Autodesk Inventor part; units mm, degrees
ref_plane "YZ Plane" through (0, 0, 0) normal (1, 0, 0) x (0, 1, 0)
ref_plane "XZ Plane" through (0, 0, 0) normal (0, 1, 0) x (-1, 0, 0)
ref_plane "XY Plane" through (0, 0, 0) normal (0, 0, 1) x (1, 0, 0)
sketch "Sketch1" plane through (0, 0, 0) normal (0, 0, 1) x (1, 0, 0)
  line L0 (-32, 32) -> (32, 32)
  line L1 (32, 32) -> (32, -32)
  line L2 (32, -32) -> (-32, -32)
  line L3 (-32, -32) -> (-32, 32)
  line L4 (-32, 32) -> (32, -32) construction
  line L5 (32, 32) -> (-32, -32) construction
  point P0 (0, 0)
  dimension "d0" = 64
  dimension "d1" = 64
extrude "Extrusion1" add sketch "Sketch1" along normal blind 3.5
sketch "Sketch2" plane through (0, 0, 3.5) normal (0, 0, 1) x (1, 0, 0)
  line L0 (-27, 27) -> (27, 27)
  line L1 (27, 27) -> (27, -27)
  line L2 (27, -27) -> (-27, -27)
  line L3 (-27, -27) -> (-27, 27)
  line L4 (-27, 27) -> (27, -27) construction
  line L5 (27, 27) -> (-27, -27) construction
  point P0 (0, 0)
  dimension "d4" = 54
  dimension "d5" = 54
extrude "Extrusion2" cut sketch "Sketch2" against normal blind 0.7
sketch "Sketch3" plane through (0, 0, 0) normal (0, 0, 1) x (1, 0, 0)
  line L0 (-32, 32) -> (-32, -32)
  line L1 (32, -32) -> (32, 32)
  line L2 (-32, -32) -> (32, -32)
  line L3 (32, -32) -> (32, 32)
  line L4 (32, 32) -> (-32, 32)
  line L5 (-32, 32) -> (-46.1421, 46.1421)
  circle A0 centre (-46.1421, 46.1421) radius 10
  line L6 (-36.4829, 43.5539) -> (-24.9289, 32)
  line L7 (32, 32) -> (-32, 32)
  line L8 (-43.5539, 36.4829) -> (-32, 24.9289)
  line L9 (32, 32) -> (46.1421, 46.1421)
  circle A1 centre (46.1421, 46.1421) radius 10
  line L10 (43.5539, 36.4829) -> (32, 24.9289)
  line L11 (36.4829, 43.5539) -> (24.9289, 32)
  line L12 (-32, -32) -> (-46.1421, -46.1421)
  circle A2 centre (-46.1421, -46.1421) radius 10
  line L13 (-36.4829, -43.5539) -> (-23.7494, -30.8205)
  line L14 (-43.5539, -36.4829) -> (-32, -24.9289)
  line L15 (32, -32) -> (46.1421, -46.1421)
  circle A3 centre (46.1421, -46.1421) radius 10
  line L16 (43.5539, -36.4829) -> (32, -24.9289)
  line L17 (36.4829, -43.5539) -> (24.9289, -32)
  point P0 (0, 0)
  point P1 (-30.7059, 37.777)
  point P2 (-24.9289, -32)
  dimension "d28" = 135
  dimension "d29" = 20
  dimension "d30" = 20
  dimension "d31" = 5
  dimension "d32" = 5
  dimension "d33" = 135
  dimension "d34" = 20
  dimension "d35" = 20
  dimension "d36" = 5
  dimension "d37" = 5
  dimension "d38" = 20
  dimension "d39" = 135
  dimension "d40" = 20
  dimension "d41" = 5
  dimension "d42" = 5
  dimension "d43" = 20
  dimension "d44" = 135
  dimension "d45" = 20
  dimension "d46" = 5
  dimension "d47" = 5
extrude "Extrusion3" add sketch "Sketch3" along normal blind 3.5 contours L5 A0 L6 L4 | L0 L8 A0 L5 | A0 | L0 L12 A2 L14 | L11 A1 L9 L4 | L2 L13 A2 L12 | A2 | L9 A1 L10 L1 | A1 | L2 L15 A3 L17 | L16 A3 L15 L1 | A3
sketch "Sketch4" plane through (0, 0, 3.5) normal (0, 0, 1) x (1, 0, 0)
  arc A0 (-36.4829, 43.5539) -> (-43.5539, 36.4829) centre (-46.1421, 46.1421) ccw
  arc A1 (43.5539, 36.4829) -> (36.4829, 43.5539) centre (46.1421, 46.1421) ccw
  arc A2 (36.4829, -43.5539) -> (43.5539, -36.4829) centre (46.1421, -46.1421) ccw
  arc A3 (-43.5539, -36.4829) -> (-36.4829, -43.5539) centre (-46.1421, -46.1421) ccw
  circle A4 centre (-46.1421, 46.1421) radius 8.25
  circle A5 centre (46.1421, 46.1421) radius 8.25
  circle A6 centre (46.1421, -46.1421) radius 8.25
  circle A7 centre (-46.1421, -46.1421) radius 8.25
  point P0 (0, 0)
  dimension "d50" = 16.5
  dimension "d51" = 16.5
  dimension "d52" = 16.5
  dimension "d53" = 16.5
extrude "Extrusion4" cut sketch "Sketch4" against normal blind 1
properties part number "holder"
Design review of the part built by this model. Coordinates are the model's own, in mm. A direction names the side the tool comes from. Round coordinates to 2 decimals unless told otherwise and drop trailing zeros. Write each loop counter-clockwise with the first axis right and the second up, starting at its lowest first coordinate (ties: lowest second). Pieces come first, ordered by that corner, then holes. Notation, with made-up numbers: (52.5, -28.75) - (94.5, -28.75) arc R13 ccw to (94.5, -21.75) - close; hole circle Ø10 at (-9, -12). An arc over 180 degrees is marked (long way). Use a Markdown table: item, result. Add a question column.
1. We need section C-C (x = 40.5). State the section outline as (y, z) points.
2. We need section B-B (y = 49.5). State the section outline as (x, z) points.
3. Mouldability with a two-part tool opening along Y and no side actions: class faces 1 (the face through (0, 32, 2)), 2 (the face through (-47.22, 54.32, 3.01)), 3 (the face through (0, -32, 2)) as +Y half, -Y half, draft (parallel to the pull), parting line (faces both ways), or undercut.
4. For faces 4 (the face through (-46, 46, 2.5)), 5 (the face through (32, 0, 2)), list the 3-axis set-ups (+Z, -Z, +X, -X, +Y, -Y) from which the entire face can be reached by the end or side of a thin tool; tool diameter is ignored.
5. Wall thickness on probe 1 along Y at (x, z) = (39, 3.35); probe 2 along X at (y, z) = (46, 0.85); probe 3 along Y at (x, z) = (-23.5, 3.35): over which ranges is each line inside the solid? List them lowest first.
6. We need section A-A (x = -6). State the section outline as (y, z) points, then the cut area to 3 significant figures.
7. We need section D-D (z = 0.7). State the section outline as (x, y) points.
8. Clearance check with flat-ended pins moving along their axes: pin 1 (1 mm diameter, centred on x = -40, z = 1, fed in from -Y); pin 2 (0.6 mm diameter, centred on x = 3.5, z = 3, fed in from -Y); pin 3 (5 mm diameter, centred on x = -43.5, y = -47, fed in from +Z). State where each tip first meets the part, or that it passes through.
Output:
| question | item | result |
|---|---|---|
| 1 | outline | (-54.4, 0) - (-33.43, 0) - (-33.43, 3.5) - (-40.12, 3.5) - (-40.12, 2.5) - (-52.16, 2.5) - (-52.16, 3.5) - (-54.4, 3.5) - close; (33.43, 0) - (54.4, 0) - (54.4, 3.5) - (52.16, 3.5) - (52.16, 2.5) - (40.12, 2.5) - (40.12, 3.5) - (33.43, 3.5) - close |
| 2 | outline | (-55.56, 0) - (-36.72, 0) - (-36.72, 3.5) - (-38.61, 3.5) - (-38.61, 2.5) - (-53.68, 2.5) - (-53.68, 3.5) - (-55.56, 3.5) - close; (36.72, 0) - (55.56, 0) - (55.56, 3.5) - (53.68, 3.5) - (53.68, 2.5) - (38.61, 2.5) - (38.61, 3.5) - (36.72, 3.5) - close |
| 3 | face 1 | +Y half |
| 3 | face 2 | undercut |
| 3 | face 3 | -Y half |
| 4 | face 4 | +Z |
| 4 | face 5 | +Z, -Z, +X |
| 5 | probe 1 | y = -53.14 to -50.27, -42.01 to -31.93, 31.93 to 42.01, 50.27 to 53.14 |
| 5 | probe 2 | x = -56.14 to -36.14, 36.14 to 56.14 |
| 5 | probe 3 | y = -32 to -27, 27 to 32 |
| 6 | outline | (-32, 0) - (32, 0) - (32, 3.5) - (27, 3.5) - (27, 2.8) - (-27, 2.8) - (-27, 3.5) - (-32, 3.5) - close |
| 6 | area | 186 mm2 |
| 7 | outline | (-43.55, -36.48) arc R10 ccw (long way) to (-36.48, -43.55) - (-24.93, -32) - (24.93, -32) - (36.48, -43.55) arc R10 ccw (long way) to (43.55, -36.48) - (32, -24.93) - (32, 24.93) - (43.55, 36.48) arc R10 ccw (long way) to (36.48, 43.55) - (24.93, 32) - (-24.93, 32) - (-36.48, 43.55) arc R10 ccw (long way) to (-43.55, 36.48) - (-32, 24.93) - (-32, -24.93) - close |
| 8 | pin 1 | stops at y = -54.4 |
| 8 | pin 2 | stops at y = -32 |
| 8 | pin 3 | stops at z = 2.5 |
